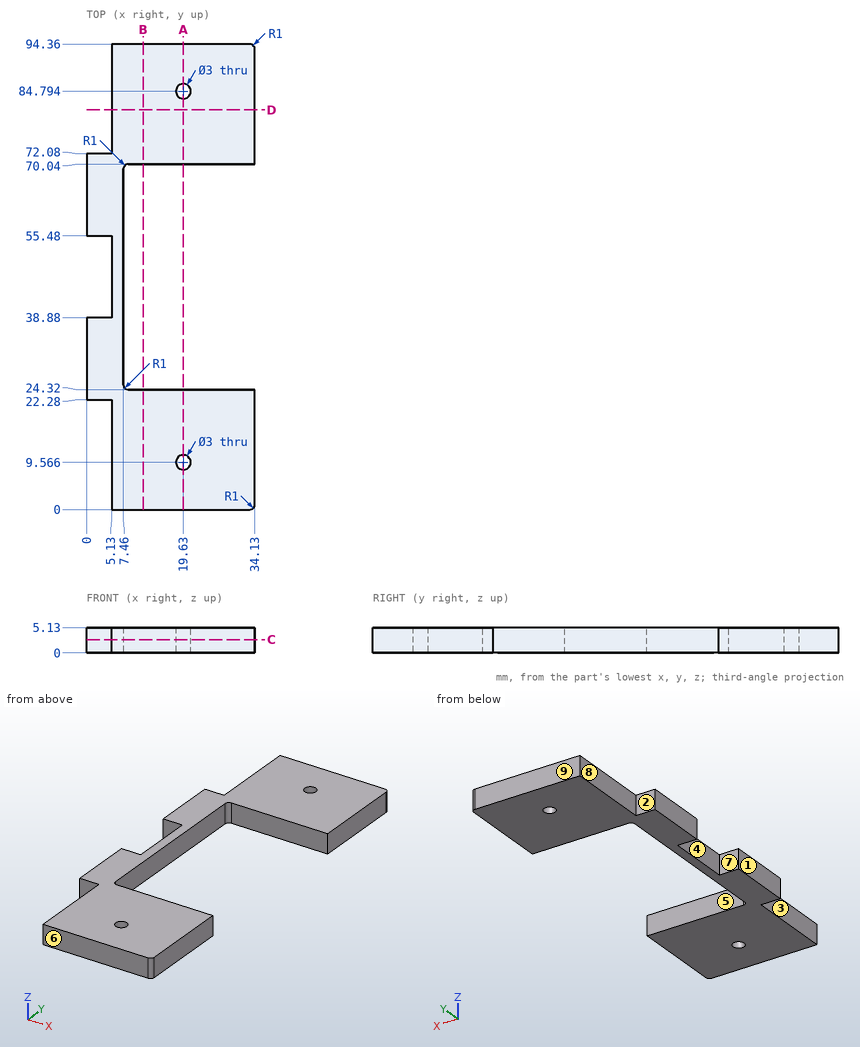
Verification items for this drawing (mm, ordinates from the low corner). A direction names the side the tool comes from. Coordinates: 2 decimals unless noted, no trailing zeros. Loops run counter-clockwise (first coordinate to the right, second up) from the corner with the lowest first, then second, coordinate; pieces in that order, holes last.
Item 1: Go/stop test with flat-tipped pins: pin 1 Ø1.5 at (x, z) = (2.5, 3) entering from -Y; pin 2 Ø2.5 at (y, z) = (41, 2.5) entering from +X; pin 3 Ø2.5 at (x, y) = (19.63, 9.566) entering from -Z; pin 4 Ø2.5 at (y, z) = (50, 2) entering from -X. Record where each tip stops, or that it passes through.
Item 2: Sectioned sample at D-D, the plane y = 81. Record the boundary of the cut face in (x, z).
Item 3: Thickness scan on line 1 (Y direction, x = 19.63, z = 3.2); line 2 (Y direction, x = 3, z = 4.7); line 3 (Y direction, x = 18.5, z = 3.1). Record the ranges inside material, lowest first.
Item 4: Sectioned sample at B-B, the plane x = 11.5. Record the boundary of the cut face in (y, z).
Item 5: Sectioned sample at A-A, the plane x = 19.63. Record the boundary of the cut face in (y, z), then the cut area to 3 significant figures.
Item 6: Release check for a two-part mould opening along Y. For the marked faces 6, 7, 8 and 9 record: released by +Y, released by -Y, zero draft, split by the parting line, or undercut.
Item 7: Sectioned sample at C-C, the plane z = 2.7. Record the boundary of the cut face in (x, y), then the cut area to 3 significant figures.
Item 8: Access from +Z, -Z, +X, -X, +Y, -Y to the whole of each face (thin tool, end or side, straight path). Record for the marked faces 1, 2, 3, 4 and 5.
Check result:
1. pin 1: stops at y = 22.28
1. pin 2: stops at x = 7.46
1. pin 3: passes through
1. pin 4: stops at x = 5.13
2. outline: (5.13, 0) - (34.13, 0) - (34.13, 5.13) - (5.13, 5.13) - close
3. line 1: y = 0 to 8.07, 11.07 to 24.32, 70.04 to 83.29, 86.29 to 94.36
3. line 2: y = 22.28 to 38.88, 55.48 to 72.08
3. line 3: y = 0 to 8.58, 10.55 to 24.32, 70.04 to 83.81, 85.78 to 94.36
4. outline: (0, 0) - (24.32, 0) - (24.32, 5.13) - (0, 5.13) - close; (70.04, 0) - (94.36, 0) - (94.36, 5.13) - (70.04, 5.13) - close
5. outline: (0, 0) - (8.07, 0) - (8.07, 5.13) - (0, 5.13) - close; (11.07, 0) - (24.32, 0) - (24.32, 5.13) - (11.07, 5.13) - close; (70.04, 0) - (83.29, 0) - (83.29, 5.13) - (70.04, 5.13) - close; (86.29, 0) - (94.36, 0) - (94.36, 5.13) - (86.29, 5.13) - close
5. area: 219 mm2
6. face 6: released by -Y
6. face 7: undercut
6. face 8: zero draft
6. face 9: released by +Y
7. outline: (0, 22.28) - (5.13, 22.28) - (5.13, 0) - (33.13, 0) arc R1 ccw to (34.13, 1) - (34.13, 24.32) - (8.46, 24.32) arc R1 cw to (7.46, 25.32) - (7.46, 69.04) arc R1 cw to (8.46, 70.04) - (34.13, 70.04) - (34.13, 93.36) arc R1 ccw to (33.13, 94.36) - (5.13, 94.36) - (5.13, 72.08) - (0, 72.08) - (0, 55.48) - (5.13, 55.48) - (5.13, 38.88) - (0, 38.88) - close; hole circle Ø3 at (19.63, 9.57); hole circle Ø3 at (19.63, 84.79)
7. area: 1,670 mm2
8. face 1: +Z, -Z, -X, +Y, -Y
8. face 2: +Z, -Z, -X, +Y
8. face 3: +Z, -Z, -X, -Y
8. face 4: +Z, -Z, -X
8. face 5: +Z, -Z, +X
